Design review of the part built by this model. Coordinates are the model's own, in mm. A direction names the side the tool comes from. Coordinates: 2 decimals unless noted, no trailing zeros. Loops run counter-clockwise (first coordinate to the right, second up) from the corner with the lowest first, then second, coordinate; pieces in that order, holes last.
Q1. Add section D-D on z = 16.5. Give the boundary of the cut face in (x, y).
Q2. Add section A-A on x = -40. Give the boundary of the cut face in (y, z), and give its area (3 significant figures).
Q3. Add section C-C on x = -80. Give the boundary of the cut face in (y, z).
Q4. Machinability: for faces 1 (the face through (-3, -38, 35)), 2 (the face through (-97.5, 3, 15)), 3 (the face through (-0.324, -42.624, 21.986)), which of the approach directions +Z, -Z, +X, -X, +Y, -Y give a long, thin tool a straight path to every point of the face, cutting with its end or side? Answer none if there is none.
Q5. Wall thickness on probe 1 along X at (y, z) = (-1.75, 5); probe 2 along Z at (x, y) = (-80, -0.5); probe 3 along Z at (x, y) = (-40, 0): over which ranges is each line inside the solid? List them lowest first.
Q6. Draft analysis for pull direction X (two halves, no side actions). For faces 4 (the face through (-95, 0, 14)), 5 (the face through (6, -48, 35)), 6 (the face through (-0.376, -47.324, 21.986)), state which applies: released by +X, released by -X, zero draft, split by the parting line, or undercut.
Q7. For P1, Ø12, axis at y = -40.5, z = 39, coming from the -X side; P2, Ø4, axis at x = -94, y = 2.5, coming from the -Z side; P3, Ø1.5, axis at x = -95, z = 12.5, coming from the +Y side, all flat-tipped, find the tip position at first contact; note any pin that passes through.
Solid Edge part; units mm, degrees
sketch "Sketch1" plane through (0, 0, 0) normal (0, -1, 0) x (1, 0, 0)
  line L0 (7, 45) -> (7, 25)
  line L1 (-32.5, 25) -> (7, 25)
  line L2 (-32.5, 5) -> (-32.5, 25)
  arc A0 (-32.5, 5) -> (-47.5, 5) centre (-40, 5) cw
  line L3 (-47.5, 25) -> (-47.5, 5)
  line L4 (-85, 25) -> (-47.5, 25)
  line L5 (-90, 20) -> (-85, 25)
  line L6 (-90, 10) -> (-90, 20)
  line L7 (-100, 10) -> (-90, 10)
  line L8 (-100, 35) -> (-100, 10)
  line L9 (-90, 45) -> (-100, 35)
  line L10 (7, 45) -> (-90, 45)
extrude "Protrusion1" add sketch "Sketch1" along normal mid plane 10
sketch "Sketch2" plane through (0, 0, 0) normal (0, -1, 0) x (1, 0, 0)
  circle A0 centre (-80, 30) radius 1.35
extrude "ExtrudedCutout_3" cut sketch "Sketch2" along normal mid plane 29.2691
hole "Hole_1" at (-40, -5, 5) direction (0, 1, 0) diameter 4.2 end up to next
fillet "Round_7" radius 20 2 edges at (-47.5, 0, 25) (-32.5, 0, 25)
sketch "Sketch3" plane through (7, 0, 30) normal (1, 0, 0) x (0, 1, 0)
  line L0 (5, 15) -> (-50, 15)
  line L1 (-50, 15) -> (-50, -11)
  line L2 (-50, -11) -> (-40, -11)
  line L3 (-40, -11) -> (-40, -5)
  line L4 (-40, -5) -> (5, -5)
  line L5 (5, -5) -> (5, 15)
  dimension "D1" = 50
  dimension "D2" = 40
extrude "ExtrudedProtrusion_3" add sketch "Sketch3" against normal blind 10
fillet "Round_8" radius 5 4 edges at (-3, -50, 32) (7, -50, 32) (-3, -40, 22) (7, -40, 22)
chamfer "Chamfer_5" distance 3.4 angle 60 1 edges at (7, -45, 19) measured on face at (-1.2333, -48.4333, 19)
fillet "Round_9" radius 20 1 edges at (7, 5, 35)
fillet "Round_10" radius 25 1 edges at (-3, -5, 35)
sketch "Sketch4" plane through (-50, 5, 17.5) normal (0, 1, 0) x (1, 0, 0)
  line L0 (-47.5, 7.5) -> (-47.5, -0.5)
  line L1 (-47.5, -0.5) -> (-42.5, -0.5)
  line L2 (-42.5, -0.5) -> (-42.5, 7.5)
  line L3 (-42.5, 7.5) -> (-47.5, 7.5)
  dimension "D1" = 42.5
  dimension "D2" = 42.5
extrude "ExtrudedCutout_5" cut sketch "Sketch4" against normal blind 5
sketch "Sketch5" plane through (-65, -5, 17.5) normal (0, -1, 0) x (1, 0, 0)
  line L0 (-25, -7.5) -> (-35, -5.9162)
  line L1 (-35, -5.9162) -> (-35, -7.5)
  line L2 (-35, -7.5) -> (-25, -7.5)
extrude "ExtrudedCutout_6" cut sketch "Sketch5" against normal blind 31.7921
properties material "PPA-CF"
Entries:
1. outline: (-100, -5) - (-90, -5) - (-90, 5) - (-92.5, 5) - (-92.5, 0) - (-97.5, 0) - (-97.5, 5) - (-100, 5) - close; (-51.14, -5) - (-28.86, -5) - (-28.86, 5) - (-51.14, 5) - close
2. outline: (-5, -2.5) - (5, -2.5) - (5, 2.9) - (-5, 2.9) - close; (-5, 7.1) - (5, 7.1) - (5, 45) - (-5, 45) - close
2. area: 433 mm2
3. outline: (-5, 25) - (5, 25) - (5, 28.65) - (-5, 28.65) - close; (-5, 31.35) - (5, 31.35) - (5, 45) - (-5, 45) - close
4. face 1: +Z, -Z, -X, -Y
4. face 2: -Z, +Y
4. face 3: -Z, -X, +Y
5. probe 1: x = -47.5 to -42.1, -37.9 to -32.5
5. probe 2: z = 25 to 28.65, 31.35 to 45
5. probe 3: z = -2.5 to 2.9, 7.1 to 45
6. face 4: undercut
6. face 5: released by +X
6. face 6: released by -X
7. P1: stops at x = -3
7. P2: stops at z = 10.32
7. P3: stops at y = 0
